```python
from build123d import *

# Parameters (mm, degrees)
F0_R     = 12
F1_DEPTH = 40
F2_R     = 9
F3_DEPTH = 40.001
F7_R     = 1
F8_DEPTH = 1


with BuildPart() as f1:
    # F0 (on Top) → F1 (new body)
    with BuildSketch(Plane.XY):
        Circle(F0_R)
    extrude(amount=F1_DEPTH)

    # F2 (on face) → F3 (cut, through all)
    with BuildSketch(Plane.XY.offset(40)):
        Circle(F2_R)
    extrude(amount=-F3_DEPTH, mode=Mode.SUBTRACT)

    # F4 (on Front) → F6 (revolve, cut)
    with BuildSketch(Plane.XZ):
        Polygon((-12, 21.60143), (-12, 20), (-10.39857, 21.60143), align=None)
    revolve(axis=Axis((0, 0, 20.635139), (0, 0, 1)), mode=Mode.SUBTRACT)

    # F7 (on face) → F8 (cut)
    with BuildSketch(Plane.XY.offset(40)):
        with Locations((0, 10.5)):
            Circle(F7_R)
    extrude(amount=-F8_DEPTH, mode=Mode.SUBTRACT)


solid = f1.part
```
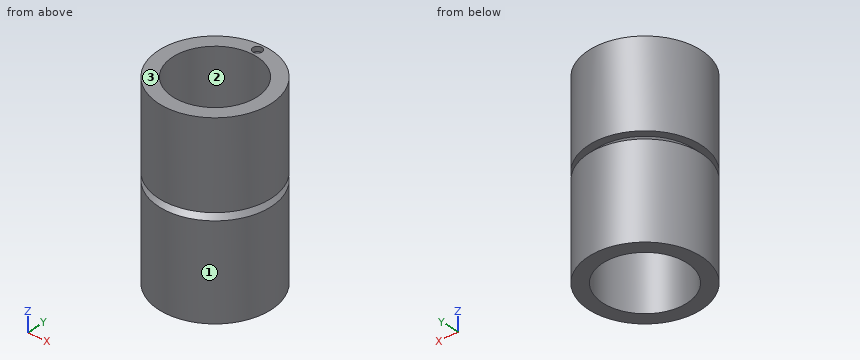
The listing builds one solid part. Answer for the finished solid, in the listing's coordinates (mm). Face numbers are marked on the shaded views. Coordinates: 2 decimals unless noted, no trailing zeros. Write each loop counter-clockwise with the first axis right and the second up, starting at its lowest first coordinate (ties: lowest second). Pieces come first, ordered by that corner, then holes. Notation, with made-up numbers: (37.5, 65.25) - (67.5, 65.25) arc R22 ccw to (67.5, 76.25) - close; hole circle Ø9 at (14.5, 45.5). An arc over 180 degrees is marked (long way). Return JSON: item names as keys, results as strings. Group by question number.
Q1. For a pull along X with two mould halves and no side action, classify the marked faces 1, 2 and 3 as +X half, -X half, draft (parallel to the pull), parting line (faces both ways), or undercut.
Q2. The part is cut by section A-A on y = 0. Write down the section's boundary in (x, z).
Q3. Find the intervals of material crossed by line 1 along Y through (x, z) = (0, 25.5); line 2 along Y through (x, z) = (-4.75, 20.5); line 3 along X through (y, z) = (4.5, 22.5), in increasing order. Write a range as [from, to].
Q4. Flat-ended cylindrical pins translate along their axes: pin 1 Ø4 at (y, z) = (3.5, 5) entering from +X; pin 2 Ø6 at (x, z) = (-3, 19) entering from +Y; pin 3 Ø2 at (x, z) = (-4.5, 18.5) entering from +Y; pin 4 Ø2 at (y, z) = (-1.5, 33) entering from -X. Find the tip coordinate at first contact, or state that the pin passes through.
Q5. The part is cut by section B-B on x = 0. Write down the section's boundary in (y, z), and give its area (3 significant figures).
Q6. The part is cut by section C-C on z = 15. Write down the section's boundary in (x, y), and give its area (3 significant figures).
Evaluation:
{
 "1": {"face 1": "parting line", "face 2": "undercut", "face 3": "draft"},
 "2": {"outline": "(-12, 0) - (-9, 0) - (-9, 40) - (-12, 40) - (-12, 21.6) - (-10.4, 21.6) - (-12, 20) - close; (9, 0) - (12, 0) - (12, 20) - (10.4, 21.6) - (12, 21.6) - (12, 40) - (9, 40) - close"},
 "3": {"line 1": "y = [-12, -9], [9, 12]", "line 2": "y = [-10.47, -7.64], [7.64, 10.47]", "line 3": "x = [-11.12, -7.79], [7.79, 11.12]"},
 "4": {"pin 1": "stops at x = 11.91", "pin 2": "stops at y = 12", "pin 3": "stops at y = 11.48", "pin 4": "stops at x = -11.99"},
 "5": {"outline": "(-12, 0) - (-9, 0) - (-9, 40) - (-12, 40) - (-12, 21.6) - (-10.4, 21.6) - (-12, 20) - close; (9, 0) - (12, 0) - (12, 20) - (10.4, 21.6) - (12, 21.6) - (12, 40) - (11.5, 40) - (11.5, 39) - (9.5, 39) - (9.5, 40) - (9, 40) - close", "area": "235 mm2"},
 "6": {"outline": "circle Ø24 at (0, 0); hole circle Ø18 at (0, 0)", "area": "198 mm2"}
}
